Print and shaded views of the part. All mm, measured from the part's lowest x, y and z. Round coordinates to 2 decimals unless told otherwise and drop trailing zeros. Write each loop counter-clockwise with the first axis right and the second up, starting at its lowest first coordinate (ties: lowest second). Pieces come first, ordered by that corner, then holes. Notation, with made-up numbers: (25, 3.25) - (50, 3.25) arc R10 cw to (50, 18.25) - close; hole circle Ø1 at (34, 31). An arc over 180 degrees is marked (long way). One line per item, written item: value.
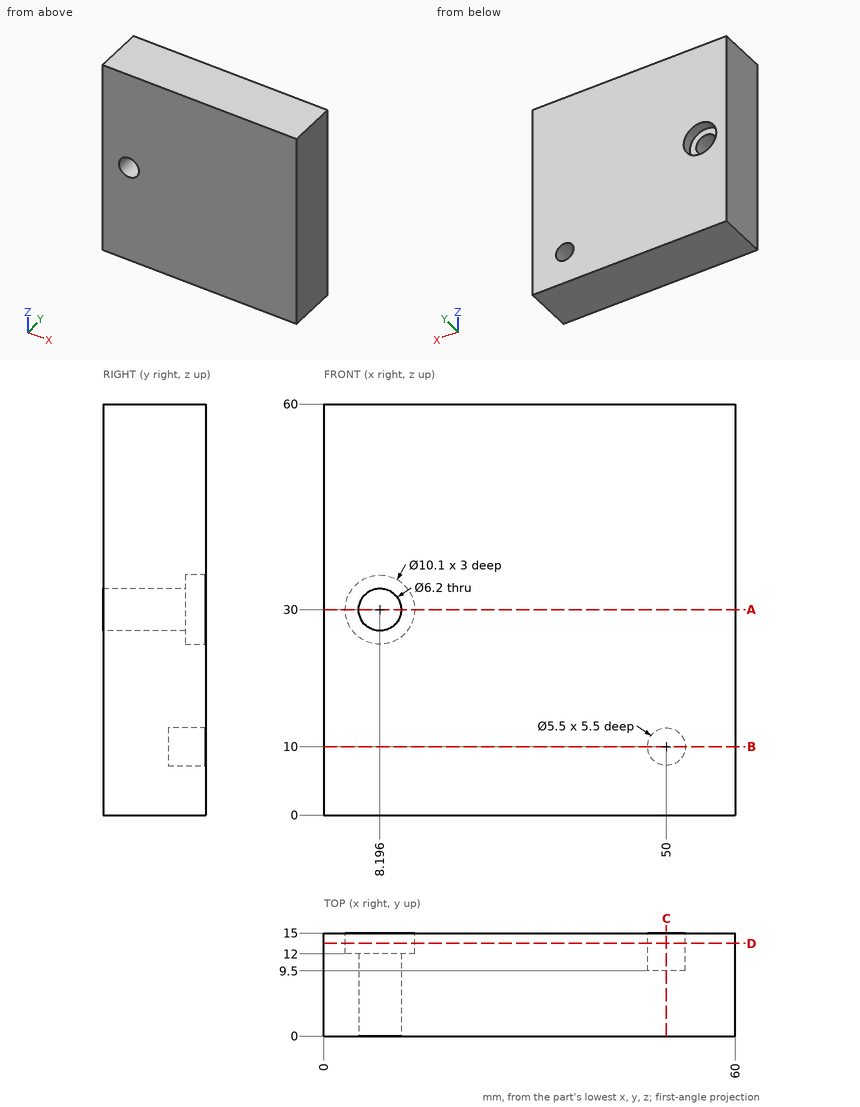
1. Wall check: probe 1 along X at (y, z) = (8.25, 30) (1 decimal); probe 2 along X at (y, z) = (13.7, 30) (1 decimal). Give the ranges that are in metal, low to high. Write a range as [from, to].
Report:
probe 1: [0, 5.1], [11.3, 60]
probe 2: [0, 3.1], [13.2, 60]
2. Drop flat-ended pins along their axis: pin 1 (3 mm diameter, centred on x = 50, z = 10, fed in from +Y); pin 2 (5 mm diameter, centred on x = 8.2, z = 30, fed in from -Y). Give the stop position or say it passes through.
Report:
pin 1: y = 9.5
pin 2: through
3. Band-saw the part on C-C on x = 50. Write the cut outline in (y, z), plus the area to 3 significant figures.
Report:
outline: (0, 0) - (15, 0) - (15, 7.25) - (9.5, 7.25) - (9.5, 12.75) - (15, 12.75) - (15, 60) - (0, 60) - close
area: 870 mm²
4. Band-saw the part on B-B on z = 10. Write the cut outline in (x, y), plus the area to 3 significant figures.
Report:
outline: (0, 0) - (60, 0) - (60, 15) - (52.75, 15) - (52.75, 9.5) - (47.25, 9.5) - (47.25, 15) - (0, 15) - close
area: 870 mm²
5. Band-saw the part on A-A on z = 30. Write the cut outline in (x, y) (1 decimal).
Report:
outline: (0, 0) - (5.1, 0) - (5.1, 12) - (3.1, 12) - (3.1, 15) - (0, 15) - close; (11.3, 0) - (60, 0) - (60, 15) - (13.2, 15) - (13.2, 12) - (11.3, 12) - close
6. Band-saw the part on D-D on y = 13.5. State how many separate pieces and enclosed holes the cut face has, plus the area to 3 significant figures.
Report:
separate pieces: 1
enclosed holes: 2
area: 3,500 mm²
